Part model, mm, in its own coordinate system. Round coordinates to 2 decimals unless told otherwise and drop trailing zeros. Write each loop counter-clockwise with the first axis right and the second up, starting at its lowest first coordinate (ties: lowest second). Pieces come first, ordered by that corner, then holes. Notation, with made-up numbers: M 77,5.25 L 126,5.25 A28 cw 126,37.25 Z; hole C 67.25,4 d9. An arc over 180 degrees is marked long. Answer as a JSON object with one key per item and string values. Group by question number.
1. Band-saw the part on B-B, the plane y = 2. Write the cut outline in (x, z).
2. Drill centre lines: line 1 (X direction, y = 5, z = 1.8); line 2 (X direction, y = 4.5, z = 5); line 3 (Y direction, x = 45, z = 3.5). Where is each one in solid material? Low to high. Write a range as from..to.
3. Band-saw the part on C-C, the plane x = 10. Write the cut outline in (y, z), plus the area to 3 significant figures.
4. Band-saw the part on D-D, the plane z = 7.75. Write the cut outline in (x, y), plus the area to 3 significant figures.
5. Two-plate mould, pull along Y, no slides. Class faces 1 (the face through (4.84, 3.74, 4.93)), 2 (the face through (38, 5, 5)), 3 (the face through (25, 0, 5)): +Y half, -Y half, draft (parallel to the pull), parting line (faces both ways), or undercut.
6. Band-saw the part on A-A, the plane z = 5. Write the cut outline in (x, y).
from build123d import *

# Parameters (mm, degrees)
ESQUISSE1_W             = 50
ESQUISSE1_H             = 10
ESQUISSE1_R             = 1.25
ESQUISSE1_R_2           = 1.75
BOSS_EXTRU_1_DEPTH      = 10
ESQUISSE2_R             = 2
ENL_V_MAT_EXTRU_1_DEPTH = 10


with BuildPart() as part:
    # Esquisse1 → Boss.-Extru.1 (new body)
    with BuildSketch(Plane.XY):
        with Locations((25, 5)):
            Rectangle(ESQUISSE1_W, ESQUISSE1_H)
        with Locations((5, 2.5)):
            Circle(ESQUISSE1_R, mode=Mode.SUBTRACT)
        with Locations((45, 2.5)):
            Circle(ESQUISSE1_R, mode=Mode.SUBTRACT)
        with Locations((40, 5)):
            Circle(ESQUISSE1_R_2, mode=Mode.SUBTRACT)
        with Locations((30, 5)):
            Circle(ESQUISSE1_R_2, mode=Mode.SUBTRACT)
        with Locations((20, 5)):
            Circle(ESQUISSE1_R_2, mode=Mode.SUBTRACT)
        with Locations((10, 5)):
            Circle(ESQUISSE1_R_2, mode=Mode.SUBTRACT)
    extrude(amount=BOSS_EXTRU_1_DEPTH)

    # Esquisse2 → Enlèv. mat.-Extru.1 (cut)
    with BuildSketch(Plane.XZ):
        with Locations(Location((40, 5, 0), (0, 0, 270))):
            Circle(ESQUISSE2_R)
        with Locations(Location((30, 5, 0), (0, 0, 270))):
            Circle(ESQUISSE2_R)
        with Locations(Location((20, 5, 0), (0, 0, 270))):
            Circle(ESQUISSE2_R)
        with Locations(Location((10, 5, 0), (0, 0, 270))):
            Circle(ESQUISSE2_R)
    extrude(amount=-ENL_V_MAT_EXTRU_1_DEPTH, mode=Mode.SUBTRACT)


solid = part.part
Worked answers:
{
 "1": {"outline": "M 0,0 L 3.85,0 L 3.85,10 L 0,10 Z; M 6.15,0 L 43.85,0 L 43.85,10 L 6.15,10 Z; M 46.15,0 L 50,0 L 50,10 L 46.15,10 Z; hole C 10,5 d4; hole C 20,5 d4; hole C 30,5 d4; hole C 40,5 d4"},
 "2": {"line 1": "x = 0..8.25, 11.75..18.25, 21.75..28.25, 31.75..38.25, 41.75..50", "line 2": "x = 0..8, 12..18, 22..28, 32..38, 42..50", "line 3": "y = 0..1.25, 3.75..10"},
 "3": {"outline": "M 0,0 L 3.25,0 L 3.25,3 L 0,3 Z; M 0,7 L 3.25,7 L 3.25,10 L 0,10 Z; M 6.75,0 L 10,0 L 10,3 L 6.75,3 Z; M 6.75,7 L 10,7 L 10,10 L 6.75,10 Z", "area": "39.0 mm^2"},
 "4": {"outline": "M 0,0 L 50,0 L 50,10 L 0,10 Z; hole C 5,2.5 d2.5; hole C 10,5 d3.5; hole C 20,5 d3.5; hole C 30,5 d3.5; hole C 40,5 d3.5; hole C 45,2.5 d2.5", "area": "452 mm^2"},
 "5": {"face 1": "undercut", "face 2": "draft", "face 3": "-Y half"},
 "6": {"outline": "M 0,0 L 8,0 L 8,10 L 0,10 Z; M 12,0 L 18,0 L 18,10 L 12,10 Z; M 22,0 L 28,0 L 28,10 L 22,10 Z; M 32,0 L 38,0 L 38,10 L 32,10 Z; M 42,0 L 50,0 L 50,10 L 42,10 Z; hole C 5,2.5 d2.5; hole C 45,2.5 d2.5"}
}
